from build123d import *

# Parameters (mm, degrees)
F0_W      = 38.1
F0_H      = 38.1
F1_DEPTH  = 38.1
F6_DEPTH  = 38.1
F8_DEPTH  = 38.1
F9_W      = 25.4
F9_H      = 7.62
F10_DEPTH = 38.1


with BuildPart() as f1:
    # F0 (on Front) → F1 (new body)
    with BuildSketch(Plane.XZ):
        with Locations((19.05, 19.05)):
            Rectangle(F0_W, F0_H)
    extrude(amount=F1_DEPTH)

    # F5 (on offset) → F6 (cut)
    with BuildSketch(Plane.YZ.offset(38.1)):
        Polygon((-31.75, 0), (-38.1, 38.1), (-38.1, 0), align=None)
        Polygon((-19.6671973258, 15.875), (-25.4, 0), (-12.7, 0), align=None)
        Polygon((-6.35, 38.1), (-31.75, 38.1), (-26.67, 16.4506547153), (-21.59, 28.575), (-16.51, 28.575), (-11.43, 17.4476634711), align=None)
        Polygon((0, 0), (0, 38.1), (-6.35, 0), align=None)
    extrude(amount=-F6_DEPTH, mode=Mode.SUBTRACT)

    # F7 (on offset) → F8 (cut)
    with BuildSketch(Plane.XZ.offset(38.1)):
        Polygon((0, 38.1), (0, 0), (6.35, 38.1), align=None)
        Polygon((25.4, 38.1), (12.7, 38.1), (19.05, 22.225), align=None)
        Polygon((11.43, 22.225), (6.35, 0), (31.75, 0), (26.67, 22.225), (21.59, 9.525), (16.51, 9.525), align=None)
        Polygon((31.75, 38.1), (38.1, 0), (38.1, 38.1), align=None)
    extrude(amount=-F8_DEPTH, mode=Mode.SUBTRACT)

    # F9 (on offset) → F10 (cut)
    with BuildSketch(Plane.XY.offset(38.1)):
        with Locations((25.4, -11.43)):
            Rectangle(F9_W, F9_H)
        with Locations((12.7, -26.67)):
            Rectangle(F9_W, F9_H)
    extrude(amount=-F10_DEPTH, mode=Mode.SUBTRACT)


solid = f1.part
Geometry: final body of the model. Coordinates: model frame, mm. A direction names the side the tool comes from. Give positions to 0.01 mm unless a question says otherwise; leave off trailing zeros. Order: outer loops, then holes, each group sorted by start corner. A loop starts at its lowest first (then second) coordinate and runs counter-clockwise, first axis right, second up. Notation, with made-up numbers: (34.25, 60) -> (42.25, 60) arc R7 cw to (42.25, 69) -> close; hole circle Ø1 at (54.25, -21.5). An arc over 180 degrees is marked (long way). Put each result on its own line as item: value.
Q1. Section D-D, the plane y = -32.5. Return loops of the section in (x, z) (3 decimals), then the cut area to 3 significant figures.
Here are the results:
outline: (0.75, 4.5) -> (7.379, 4.5) -> (11.43, 22.225) -> (16.51, 9.525) -> (21.59, 9.525) -> (26.67, 22.225) -> (30.721, 4.5) -> (37.35, 4.5) -> (31.75, 38.1) -> (25.4, 38.1) -> (19.05, 22.225) -> (12.7, 38.1) -> (6.35, 38.1) -> close
area: 728 mm^2
Q2. Section C-C, the plane z = 24. Count the separate pieces of the cut face and the enclosed holes in it, then the cut area to 3 significant figures.
Here are the results:
separate pieces: 6
enclosed holes: 0
area: 570 mm^2
Q3. Material intervals for L1, parallel to Y at x = 35, z = 8.5; L2, parallel to Y at x = 4, z = 21.5; L3, parallel to X at y = -2, z = 28, sorted ascending.
Here are the results:
L1: y = -33.17 to -22.33, -16.43 to -15.24, -7.62 to -4.93
L2: y = -35.33 to -30.48, -22.86 to -13.28, -10.43 to -2.77
L3: x = 4.67 to 16.74, 21.36 to 33.43
Q4. Section B-B, the plane x = 3.5. Return loops of the section in (y, z) (3 decimals).
Here are the results:
outline: (-35.25, 21) -> (-31.75, 0) -> (-30.48, 0) -> (-30.48, 21) -> close; (-22.86, 7.034) -> (-19.667, 15.875) -> (-12.7, 0) -> (-6.35, 0) -> (-2.85, 21) -> (-10.556, 21) -> (-11.43, 17.448) -> (-13.052, 21) -> (-22.86, 21) -> close
Q5. Pin query (flat end, axial travel): pin 1 (0.8 mm diameter, centred on x = 18.5, y = -16, fed in from -Z) (3 decimals); pin 2 (0.8 mm diameter, centred on y = -24.5, z = 21, fed in from -X); pin 3 (8 mm diameter, centred on x = 30, y = -20.5, fed in from -Z); pin 4 (2 mm diameter, centred on x = 27.5, z = 9.5, fed in from -Y). Return the tip coordinate at first contact, or that it passes through.
Here are the results:
pin 1: stops at z = 9.525
pin 2: stops at x = 25.4
pin 3: stops at z = 2.91
pin 4: passes through
Q6. Section A-A, the plane x = 36. Return loops of the section in (y, z), then the cut area to 3 significant figures.
Here are the results:
outline: (-33.85, 12.6) -> (-31.75, 0) -> (-25.4, 0) -> (-20.85, 12.6) -> close; (-18.23, 12.6) -> (-15.24, 5.79) -> (-15.24, 12.6) -> close; (-7.62, 0) -> (-6.35, 0) -> (-4.25, 12.6) -> (-7.62, 12.6) -> close
area: 161 mm^2
Q7. Reachability of faces 1 (the face through (10.222, -31.124, 35.432)), 2 (the face through (13, -30.48, 20)), 3 (the face through (28.68, -5.72, 13.43)), 4 (the face through (22.2, -4.7, 30.1)), 5 (the face through (19.121, -20.543, 13.45)) from +Z, -Z, +X, -X, +Y, -Y: full face, straight path, thin tool, end or side. Return the list, or none.
Here are the results:
face 1: +Z, +X, -X
face 2: +Z, -Z, -X
face 3: -Z, +Y, -Y
face 4: +Z, +Y, -Y
face 5: -Z, +X, -X
Q8. Draft query along Y for faces 6 (the face through (19.32, -3.13, 19.32)), 7 (the face through (8.733, -14.006, 23.089)), 8 (the face through (3.836, -33.497, 23.017)). Return one class per face: released by +Y, released by -Y, zero draft, split by the parting line, or undercut.
Here are the results:
face 6: released by +Y
face 7: undercut
face 8: zero draft
